```python
from build123d import *

# Parameters (mm, degrees)
SKETCH1_R           = 19
SKETCH1_W           = 36.78
SKETCH1_H           = 15
BOSS_EXTRUDE1_DEPTH = 15
BOSS_EXTRUDE4_DEPTH = 5


with BuildPart() as part:
    # Sketch1 → Boss-Extrude1 (new body)
    with BuildSketch(Plane.XY):
        with BuildLine():
            Line((-18.39, -12.5), (18.39, -12.5))
            ThreePointArc((18.39, -12.5), (21.925533906, -11.035533906), (23.39, -7.5))
            Line((23.39, -7.5), (23.996791899, 29.607599001))
            ThreePointArc((23.996791899, 29.607599001), (0, 54), (-23.996791899, 29.607599001))
            Line((-23.996791899, 29.607599001), (-23.39, -7.5))
            ThreePointArc((-23.39, -7.5), (-21.925533906, -11.035533906), (-18.39, -12.5))
        make_face()
        with Locations((0, 30)):
            Circle(SKETCH1_R, mode=Mode.SUBTRACT)
        Rectangle(SKETCH1_W, SKETCH1_H, mode=Mode.SUBTRACT)
    extrude(amount=BOSS_EXTRUDE1_DEPTH)

    # Sketch13 → Boss-Extrude4 (add)
    with BuildSketch(Plane.XY.offset(15)):
        with BuildLine():
            Line((-23.996791899, 29.607599001), (-23.39, -7.5))
            ThreePointArc((-23.39, -7.5), (-21.901669041, -11.011669041), (-18.39, -12.5))
            Line((-18.39, -12.5), (18.39, -12.5))
            ThreePointArc((18.39, -12.5), (21.925533906, -11.035533906), (23.39, -7.5))
            Line((23.39, -7.5), (23.996791899, 29.607599001))
            ThreePointArc((23.996791899, 29.607599001), (0, 54), (-23.996791899, 29.607599001))
        make_face()
        Polygon((-18.39, -7.5), (-18.39, 7.5), (0, 7.5), (18.39, 7.5), (18.39, -7.5), align=None, mode=Mode.SUBTRACT)
    extrude(amount=BOSS_EXTRUDE4_DEPTH)


solid = part.part
```
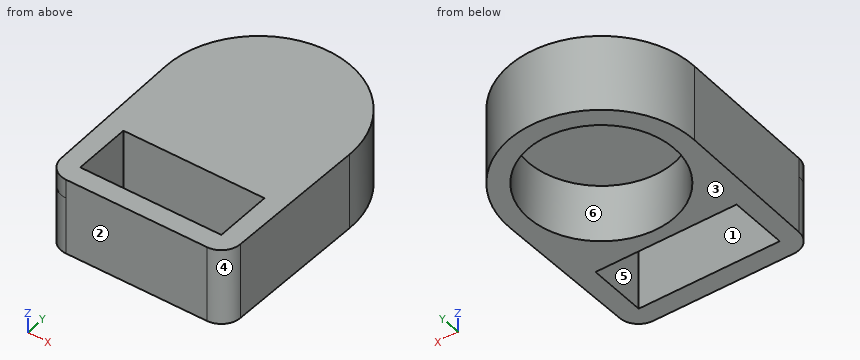
Source: CAD feature listing. Evaluate the final solid. Frame: model axes, mm. Face numbers are marked on the shaded views. A direction names the side the tool comes from. Round coordinates to 2 decimals unless told otherwise and drop trailing zeros. Loops run counter-clockwise (first coordinate to the right, second up) from the corner with the lowest first, then second, coordinate; pieces in that order, holes last.
1. Mould query, pull axis Y, two halves, no side actions, for the marked faces 1, 2 and 3. Classes: released by +Y, released by -Y, zero draft, split by the parting line, or undercut.
2. Access query for the marked faces 4, 5 and 6. Directions: +Z, -Z, +X, -X, +Y, -Y. A direction counts if a zero-diameter tool reaches every point of the face in a straight line with its end or side. Return the directions, or none.
3. Section query D-D on y = 42. Output: boundary loops of the cut face in (x, z), and give its area (3 significant figures).
4. Ray query, L1, parallel to Z at x = -14, y = 37.5; L2, parallel to Y at x = 3.5, z = 8.5; L3, parallel to Y at x = -3, z = 5. Return the intervals inside material, ascending.
5. Section query B-B on x = 0. Output: boundary loops of the cut face in (y, z).
6. Contact query for flat-ended pins moving along their axis: pin 1 (4 mm diameter, centred on x = 6, y = 16, fed in from -Z); pin 2 (1.5 mm diameter, centred on x = 12, z = 13, fed in from +Y); pin 3 (8 mm diameter, centred on x = 8.5, z = 9.5, fed in from +Y). Output: stop coordinate, or through.
Answers below:
1. face 1: undercut
1. face 2: released by -Y
1. face 3: zero draft
2. face 4: +Z, -Z, +X, -Y
2. face 5: +Z, -Z
2. face 6: -Z
3. outline: (-20.78, 0) - (-14.73, 0) - (-14.73, 15) - (14.73, 15) - (14.73, 0) - (20.78, 0) - (20.78, 20) - (-20.78, 20) - close
3. area: 389 mm2
4. L1: z = 15 to 20
4. L2: y = -12.5 to -7.5, 7.5 to 11.33, 48.67 to 53.74
4. L3: y = -12.5 to -7.5, 7.5 to 11.24, 48.76 to 53.81
5. outline: (-12.5, 0) - (-7.5, 0) - (-7.5, 20) - (-12.5, 20) - close; (7.5, 0) - (11, 0) - (11, 15) - (49, 15) - (49, 0) - (54, 0) - (54, 20) - (7.5, 20) - close
6. pin 1: stops at z = 15
6. pin 2: stops at y = 51.2
6. pin 3: stops at y = 53.57
